from build123d import *

# Parameters (mm, degrees)
BOSS_EXTRUDE1_DEPTH = 8
CUT_EXTRUDE1_DEPTH  = 8
CUT_EXTRUDE2_DEPTH  = 8
CHAMFER1_SIZE       = 1


with BuildPart() as part:
    # Sketch1 → Boss-Extrude1 (new body)
    with BuildSketch(Plane(origin=(0, 0, 0), x_dir=(0, 0, -1), z_dir=(1, 0, 0))):
        Polygon((0, 0), (25, 0), (25, 30), (20, 30), (20, 3), (0, 3), align=None)
    extrude(amount=BOSS_EXTRUDE1_DEPTH)

    # Sketch3 → Cut-Extrude1 (cut)
    with BuildSketch(Plane(origin=(0, 3, 0), x_dir=(1, 0, 0), z_dir=(0, 1, 0))):
        with BuildLine():
            Line((1.95, 4), (1.95, 16))
            ThreePointArc((1.95, 16), (4, 18.05), (6.05, 16))
            Line((6.05, 16), (6.05, 4))
            ThreePointArc((6.05, 4), (4, 1.95), (1.95, 4))
        make_face()
    extrude(amount=-CUT_EXTRUDE1_DEPTH, mode=Mode.SUBTRACT)

    # Sketch4 → Cut-Extrude2 (cut)
    with BuildSketch(Plane.XY.offset(-20)):
        with BuildLine():
            Line((6.05, 26), (6.05, 8))
            ThreePointArc((6.05, 8), (4, 5.95), (1.95, 8))
            Line((1.95, 8), (1.95, 26))
            ThreePointArc((1.95, 26), (4, 28.05), (6.05, 26))
        make_face()
    extrude(amount=-CUT_EXTRUDE2_DEPTH, mode=Mode.SUBTRACT)

    # Chamfer1
    chamfer1_edges = [part.edges().sort_by_distance(p)[0] for p in [
        (4, 3, -20),
    ]]
    chamfer(chamfer1_edges, length=CHAMFER1_SIZE)


solid = part.part
Geometry check sheet. Reference: the model listing, model coordinates, mm. A direction names the side the tool comes from. Coordinates: 2 decimals unless noted, no trailing zeros. Order: outer loops, then holes, each group sorted by start corner. A loop starts at its lowest first (then second) coordinate and runs counter-clockwise, first axis right, second up. Notation, with made-up numbers: (-19, -26.5) -> (25, -26.5) arc R11 ccw to (25, -7.5) -> close; hole circle Ø3 at (18, 11). An arc over 180 degrees is marked (long way). Use a Markdown table: item, result. Add a question column.
1. Cross-section at C-C (y = 13). Enter the section's corners in (x, z), and give its area (3 significant figures).
2. Go/stop test with a flat-tipped pin: pin 1 Ø1.5 at (x, y) = (3, 24.5) entering from -Z. Record where the tip stops, or that it passes through.
3. Cross-section at D-D (z = -23.5). Enter the section's corners in (x, y), and give its area (3 significant figures).
4. Mould release check, pull along Y, two halves, no side actions. Record for faces 4 (the face through (6.05, 17, -22)), 5 (the face through (7, 0, -12)), 6 (the face through (7, 17, -20)), 7 (the face through (3.95, 28.05, -22.46)): pulls with the +Y half, pulls with the -Y half, needs draft (parallel to the pull), parting line crosses it, or undercut.
5. Cross-section at B-B (z = -15.5). Enter the section's corners in (x, y), and give its area (3 significant figures).
6. Set-up check for faces 1 (the face through (3.95, 1.52, -18.05)), 2 (the face through (4.05, 5.95, -22.46)), 3 (the face through (7, 3, -10)): record each of +Z, -Z, +X, -X, +Y, -Y from which the full face is reachable in a straight line by a thin tool's end or side.
7. Material ranges on L1, parallel to X at y = 12.5, z = -21; L2, parallel to Y at x = 4, z = -20.25, recorded low to high.
8. Cross-section at A-A (x = 4). Enter the section's corners in (y, z), and give its area (3 significant figures).
Filled sheet:
| question | item | result |
|---|---|---|
| 1 | outline | (0, -25) -> (1.95, -25) -> (1.95, -20) -> (0, -20) -> close; (6.05, -25) -> (8, -25) -> (8, -20) -> (6.05, -20) -> close |
| 1 | area | 19.5 mm2 |
| 2 | pin 1 | through |
| 3 | outline | (0, 0) -> (8, 0) -> (8, 30) -> (0, 30) -> close; hole (1.95, 8) arc R2.05 ccw to (6.05, 8) -> (6.05, 26) arc R2.05 ccw to (1.95, 26) -> close |
| 3 | area | 153 mm2 |
| 4 | face 4 | undercut |
| 4 | face 5 | pulls with the -Y half |
| 4 | face 6 | needs draft |
| 4 | face 7 | undercut |
| 5 | outline | (0, 0) -> (1.95, 0) -> (1.95, 3) -> (0, 3) -> close; (6.05, 0) -> (8, 0) -> (8, 3) -> (6.05, 3) -> close |
| 5 | area | 11.7 mm2 |
| 6 | face 1 | +Y, -Y |
| 6 | face 2 | +Z, -Z |
| 6 | face 3 | +Z, +X, -X, +Y |
| 7 | L1 | 0 to 1.95, 6.05 to 8 |
| 7 | L2 | 0 to 5.95, 28.05 to 30 |
| 8 | outline | (0, -25) -> (5.95, -25) -> (5.95, -20) -> (4, -20) -> (3, -19) -> (3, -18.05) -> (0, -18.05) -> close; (0, -1.95) -> (3, -1.95) -> (3, 0) -> (0, 0) -> close; (28.05, -25) -> (30, -25) -> (30, -20) -> (28.05, -20) -> close |
| 8 | area | 51.7 mm2 |
